Can you work these out from the drawing? Everything is in mm from the part's minimum corner. Give positions to 0.01 mm unless a question says otherwise; leave off trailing zeros. Order: outer loops, then holes, each group sorted by start corner. A loop starts at its lowest first (then second) coordinate and runs counter-clockwise, first axis right, second up. Notation, with made-up numbers: (61, 50.5) - (88, 50.5) arc R5 ccw to (88, 54.5) - close; hole circle Ø8 at (18, -32.75). An arc over 180 degrees is marked (long way). One line per question, with ' | ' between items.
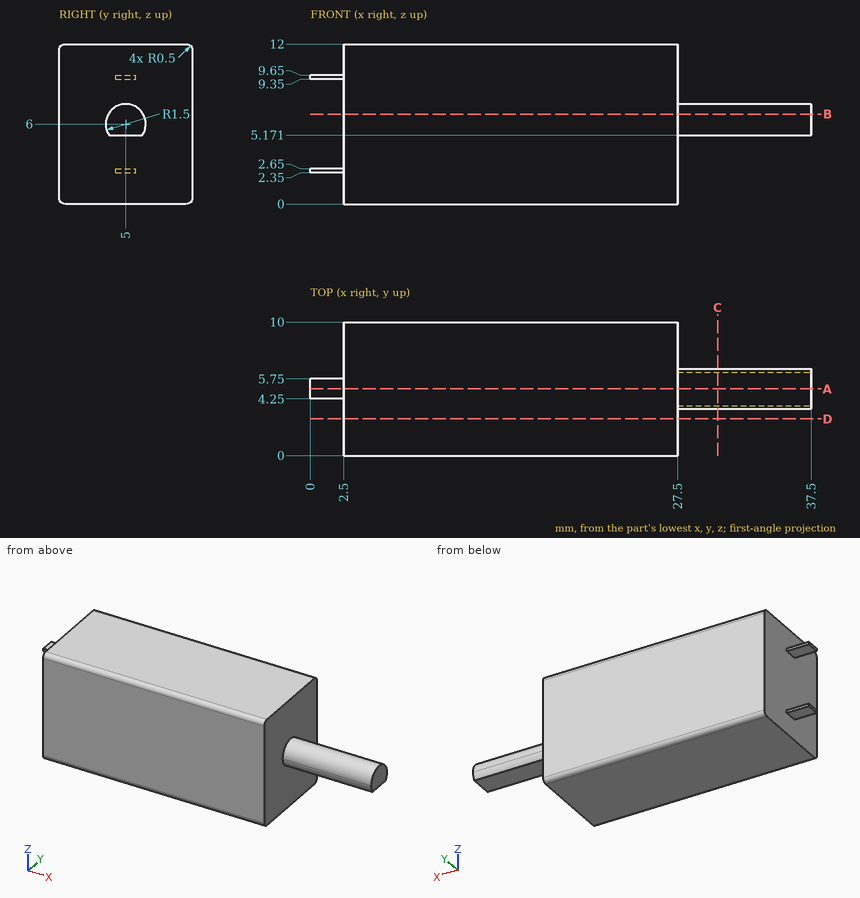
(1) Imagine slicing it at C-C (x = 30.5). List the corners of the cut face in (y, z) for me, and give its area (3 significant figures).
Answer below:
outline: (3.75, 5.17) - (6.25, 5.17) arc R1.5 ccw (long way) to start | area: 5.89 mm^2
(2) Will these pins go through, and if not, where does the flat tip stop? pin 1 (3 mm diameter, centred on x = 7, y = 2.5, fed in from -Z); pin 2 (1.2 mm diameter, centred on x = 1, y = 5, fed in from -Z); pin 3 (2 mm diameter, centred on x = 33.5, y = 5.5, fed in from -Z); pin 4 (1.6 mm diameter, centred on x = 1.5, y = 4.5, fed in from +Z).
Answer below:
pin 1: z = 0 | pin 2: z = 2.35 | pin 3: z = 5.17 | pin 4: z = 9.65
(3) If I drill on line 1 (X direction, y = 7, z = 2); line 2 (Z direction, x = 36.5, y = 5.25), over which ranges is the centre line in solid material (lowest first)?
Answer below:
line 1: 2.5 to 27.5 | line 2: 5.17 to 7.48
(4) Imagine slicing it at B-B (z = 6.75). List the corners of the cut face in (x, y) for me.
Answer below:
outline: (2.5, 0) - (27.5, 0) - (27.5, 3.7) - (37.5, 3.7) - (37.5, 6.3) - (27.5, 6.3) - (27.5, 10) - (2.5, 10) - close
(5) Imagine slicing it at D-D (y = 2.75). List the corners of the cut face in (x, z) for me.
Answer below:
outline: (2.5, 0) - (27.5, 0) - (27.5, 12) - (2.5, 12) - close
(6) Imagine slicing it at A-A (y = 5). List the corners of the cut face in (x, z) for me.
Answer below:
outline: (0, 2.35) - (2.5, 2.35) - (2.5, 0) - (27.5, 0) - (27.5, 5.17) - (37.5, 5.17) - (37.5, 7.5) - (27.5, 7.5) - (27.5, 12) - (2.5, 12) - (2.5, 9.65) - (0, 9.65) - (0, 9.35) - (2.5, 9.35) - (2.5, 2.65) - (0, 2.65) - close
